```python
from build123d import *

# Parameters (mm, degrees)
SKETCH1_R           = 25
BOSS_EXTRUDE1_DEPTH = 7.5
SKETCH2_R           = 5
BOSS_EXTRUDE2_DEPTH = 12
BOSS_EXTRUDE3_DEPTH = 5
SKETCH4_R           = 10
BOSS_EXTRUDE4_DEPTH = 2


with BuildPart() as part:
    # Sketch1 → Boss-Extrude1 (new, symmetric)
    with BuildSketch(Plane(origin=(0, 0, 0), x_dir=(0, 0, -1), z_dir=(1, 0, 0))):
        Circle(SKETCH1_R)
    extrude(amount=BOSS_EXTRUDE1_DEPTH, both=True)

    # Sketch2 → Boss-Extrude2 (add)
    with BuildSketch(Plane(origin=(7.5, 0, 0), x_dir=(0, 0, -1), z_dir=(1, 0, 0))):
        Circle(SKETCH2_R)
    extrude(amount=BOSS_EXTRUDE2_DEPTH)

    # Sketch3 → Boss-Extrude3 (add)
    with BuildSketch(Plane.ZY.offset(7.5)):
        with BuildLine():
            Line((2.5, 24.874685928), (2.5, -24.874685928))
            ThreePointArc((2.5, -24.874685928), (0, -25), (-2.5, -24.874685928))
            Line((-2.5, -24.874685928), (-2.5, 24.874685928))
            ThreePointArc((-2.5, 24.874685928), (0, 25), (2.5, 24.874685928))
        make_face()
    extrude(amount=BOSS_EXTRUDE3_DEPTH)

    # Sketch4 → Boss-Extrude4 (add)
    with BuildSketch(Plane(origin=(7.5, 0, 0), x_dir=(0, 0, -1), z_dir=(1, 0, 0))):
        Circle(SKETCH4_R)
    extrude(amount=BOSS_EXTRUDE4_DEPTH)


solid = part.part
```
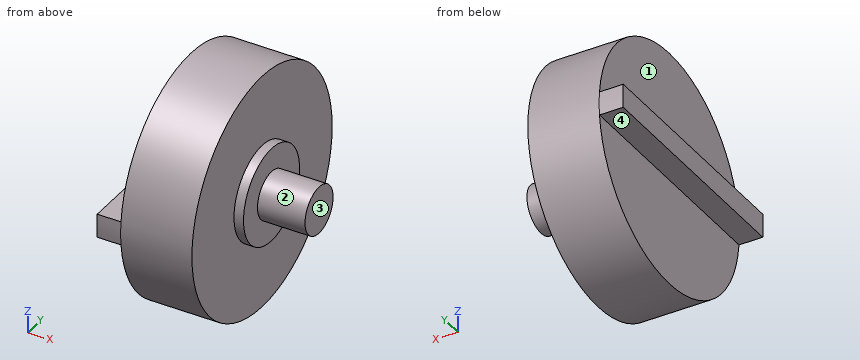
Can you work these out from the model? Positions are in its coordinate system, mm. Face numbers are marked on the shaded views. A direction names the side the tool comes from. Coordinates: 2 decimals unless noted, no trailing zeros. Loops run counter-clockwise (first coordinate to the right, second up) from the corner with the lowest first, then second, coordinate; pieces in that order, holes last. Notation, with made-up numbers: (-22, 69) - (9, 69) arc R27 ccw to (9, 96) - close; hole circle Ø8 at (-19, -25). An arc over 180 degrees is marked (long way). Answer as CSV lines item,"result". Start each with the question number.
1) Suppose I cut it at D-D (z = -20). Please give me the cut outline in (x, y).
2) For pin 1 (12 mm diameter, centred on x = 1, y = -9, fed in from +Z); pin 2 (4 mm diameter, centred on x = -10, y = 0.5, fed in from -Z); pin 3 (2 mm diameter, centred on y = -15, z = -14, fed in from -X), each with a flat end and sliding along its axis, tell me the tip position at first contact or that it passes through.
3) Suppose I cut it at A-A (y = 0). Please give me the cut outline in (x, z), plus the area to 3 significant figures.
4) I need wall thicknesses on line 1 (X direction, y = -12, z = -11.5); line 2 (Y direction, x = 14, z = 0); line 3 (Z direction, x = -9, y = 14). Which ranges of each line are inside material? Lowest first, please. Write a range as from..to.
5) Suppose I cut it at C-C (x = 5). Please give me the cut outline in (y, z).
6) Suppose I cut it at B-B (z = 0). Please give me the cut outline in (x, y).
7) Which directions (+Z, -Z, +X, -X, +Y, -Y) give clear straight access to the entire face, cutting with the end or side of a thin tool? Please do the marked faces 1, 2, 3 and 4.
Check result:
1,outline,"(-7.5, -15) - (7.5, -15) - (7.5, 15) - (-7.5, 15) - close"
2,pin 1,"stops at z = 24.82"
2,pin 2,"stops at z = -2.5"
2,pin 3,"stops at x = -7.5"
3,outline,"(-12.5, -2.5) - (-7.5, -2.5) - (-7.5, -25) - (7.5, -25) - (7.5, -10) - (9.5, -10) - (9.5, -5) - (19.5, -5) - (19.5, 5) - (9.5, 5) - (9.5, 10) - (7.5, 10) - (7.5, 25) - (-7.5, 25) - (-7.5, 2.5) - (-12.5, 2.5) - close"
3,area,"915 mm²"
4,line 1,"x = -7.5..7.5"
4,line 2,"y = -5..5"
4,line 3,"z = -2.5..2.5"
5,outline,"circle Ø50 at (0, 0)"
6,outline,"(-12.5, -25) - (7.5, -25) - (7.5, -10) - (9.5, -10) - (9.5, -5) - (19.5, -5) - (19.5, 5) - (9.5, 5) - (9.5, 10) - (7.5, 10) - (7.5, 25) - (-12.5, 25) - close"
7,face 1,"+Z, -X, +Y, -Y"
7,face 2,"+X"
7,face 3,"+Z, -Z, +X, +Y, -Y"
7,face 4,"-Z, -X, +Y, -Y"
